```python
from build123d import *

# Parameters (mm, degrees)
F0_W     = 700
F0_H     = 700
F1_DEPTH = 2000
F2_T     = -16
F3_R     = 50
F4_R     = 34


# Not quite as in the source:
# - a feature names something its author has since deleted; it is built from what else it names


with BuildPart() as f1:
    # F0 (on Top) → F1 (new body)
    with BuildSketch(Plane.XY):
        with Locations((-350, -350)):
            Rectangle(F0_W, F0_H)
    extrude(amount=F1_DEPTH)

    # F2
    f2_openings = [f1.faces().sort_by_distance(p)[0] for p in [
        (-350, 0, 1000),
        (-350, -350, 2000),
        (-350, -350, 0),
    ]]
    offset(amount=F2_T, openings=f2_openings)

    # F3
    f3_edges = [f1.edges().sort_by_distance(p)[0] for p in [
        (0, -700, 1000),
    ]]
    fillet(f3_edges, radius=F3_R)

    # F4
    f4_edges = [f1.edges().sort_by_distance(p)[0] for p in [
        (-16, -684, 1000),
    ]]
    fillet(f4_edges, radius=F4_R)


solid = f1.part
```
Check sheet for the modelled part. Datum: model origin and axes. Units: mm. A direction names the side the tool comes from. Round coordinates to 2 decimals unless told otherwise and drop trailing zeros. Order: outer loops, then holes, each group sorted by start corner. A loop starts at its lowest first (then second) coordinate and runs counter-clockwise, first axis right, second up. Notation, with made-up numbers: (31, 12.5) -> (52, 12.5) arc R23 cw to (52, 49.5) -> close; hole circle Ø10 at (65.25, 35). An arc over 180 degrees is marked (long way). One line per item, written item: value. Start each with the question number.
Q1. Cross-section at C-C (x = -98.5). Record the boundary of the cut face in (y, z).
Q2. Thickness scan on line 1 (X direction, y = -312, z = 710); line 2 (Y direction, x = -242, z = 1458.5); line 3 (Y direction, x = -46.5, z = 1280). Record the ranges inside material, lowest first.
Q3. Cross-section at B-B (z = 872.5). Record the boundary of the cut face in (x, y).
Q4. Set-up check for faces 5 (the face through (-684, -347, 986)), 6 (the face through (-352, -685, 0)): record each of +Z, -Z, +X, -X, +Y, -Y from which the full face is reachable in a straight line by a thin tool's end or side.
Q5. Gauge pin test, flat end, axial feed: pin 1 Ø1 at (x, z) = (-207, 477.5) entering from +Y. Record the tip position at first contact, or that the pin passes through.
Q6. Cross-section at A-A (y = -214). Record the boundary of the cut face in (x, z), and give its area (3 significant figures).
Q7. Mould release check, pull along X, two halves, no side actions. Record for faces 1 (the face through (-371, -684, 986)), 2 (the face through (-700, -355, 986)), 3 (the face through (0, -330, 986)), 4 (the face through (-380, -700, 986)): pulls with the +X half, pulls with the -X half, needs draft (parallel to the pull), parting line crosses it, or undercut.
Completed:
1. outline: (-700, 0) -> (-684, 0) -> (-684, 2000) -> (-700, 2000) -> close
2. line 1: x = -700 to -684, -16 to 0
2. line 2: y = -700 to -684
2. line 3: y = -699.88 to -683.82
3. outline: (-700, -700) -> (-50, -700) arc R50 ccw to (0, -650) -> (0, 0) -> (-16, 0) -> (-16, -650) arc R34 cw to (-50, -684) -> (-684, -684) -> (-684, 0) -> (-700, 0) -> close
4. face 5: +Z, -Z, +Y
4. face 6: -Z, +X, -X, +Y, -Y
5. pin 1: stops at y = -684
6. outline: (-700, 0) -> (-684, 0) -> (-684, 2000) -> (-700, 2000) -> close; (-16, 0) -> (0, 0) -> (0, 2000) -> (-16, 2000) -> close
6. area: 64,000 mm²
7. face 1: undercut
7. face 2: pulls with the -X half
7. face 3: pulls with the +X half
7. face 4: needs draft
